Check sheet for the modelled part. Datum: model origin and axes. Units: mm. A direction names the side the tool comes from. Round coordinates to 2 decimals unless told otherwise and drop trailing zeros. Order: outer loops, then holes, each group sorted by start corner. A loop starts at its lowest first (then second) coordinate and runs counter-clockwise, first axis right, second up. Notation, with made-up numbers: M 58.25,73.25 L 84.25,73.25 A18 cw 84.25,82.25 Z; hole C 44.5,23.5 d1. An arc over 180 degrees is marked long. One line per item, written item: value. Start each with the question number.
(1) Cross-section at D-D, the plane y = -17. Enter the section's corners in (x, z), and give its area (3 significant figures).
(2) Release check for a two-part mould opening along X. For faces 3 (the face through (-13, -4, -7)), 4 (the face through (0, 17.75, -7)), 5 (the face through (20, 0, 2)) record: released by +X, released by -X, zero draft, split by the parting line, or undercut.
(3) Depth check by flat-ended pin: pin 1 Ø4 at (x, z) = (-1.5, -7) entering from +Y; pin 2 Ø3.5 at (y, z) = (-8.5, -9.5) entering from +X; pin 3 Ø2 at (y, z) = (2.5, -7.5) entering from -X. Enter the tip coordinate at first touch or a pass-through.
(4) Cross-section at C-C, the plane x = -1. Enter the section's corners in (y, z), and give its area (3 significant figures).
(5) Cross-section at A-A, the plane z = -6.5. Enter the section's corners in (x, y), and give its area (3 significant figures).
(6) Access from +Z, -Z, +X, -X, +Y, -Y to the whole of each face (thin tool, end or side, straight path). Record for faces 1 (the face through (10, 15.25, -7)), 2 (the face through (19.43, -19.4, 1.97)).
(7) Thickness scan on L1, parallel to Y at x = 15, z = -9.5; L2, parallel to X at y = -6, z = -1.5. Record the ranges inside material, lowest first.
(8) Cross-section at B-B, the plane y = 7.5. Enter the section's corners in (x, z), and give its area (3 significant figures).
from build123d import *

# Parameters (mm, degrees)
P_IDAT_VYSUNUT_M1_DEPTH = 4
SKICA2_W                = 30.5
SKICA2_H                = 30.5
SKICA2_W_2              = 4
SKICA2_H_2              = 4
P_IDAT_VYSUNUT_M2_DEPTH = 15


with BuildPart() as part:
    # Skica1 → Přidat vysunutím1 (new body)
    with BuildSketch(Plane.XY):
        with BuildLine():
            Line((-18, 20), (18, 20))
            ThreePointArc((18, 20), (19.414213562, 19.414213562), (20, 18))
            Line((20, 18), (20, -18))
            ThreePointArc((20, -18), (19.414213562, -19.414213562), (18, -20))
            Line((18, -20), (-18, -20))
            ThreePointArc((-18, -20), (-19.414213562, -19.414213562), (-20, -18))
            Line((-20, -18), (-20, 18))
            ThreePointArc((-20, 18), (-19.414213562, 19.414213562), (-18, 20))
        make_face()
    extrude(amount=P_IDAT_VYSUNUT_M1_DEPTH)

    # Skica2 → Přidat vysunutím2 (add)
    with BuildSketch(Plane(origin=(0, 0, 0), x_dir=(-1, 0, 0), z_dir=(0, 0, -1))):
        with BuildLine():
            ThreePointArc((-17.75, 15.75), (-17.164213562, 17.164213562), (-15.75, 17.75))
            Line((-15.75, 17.75), (15.75, 17.75))
            ThreePointArc((15.75, 17.75), (17.164213562, 17.164213562), (17.75, 15.75))
            Line((17.75, 15.75), (17.75, -15.75))
            ThreePointArc((17.75, -15.75), (17.164213562, -17.164213562), (15.75, -17.75))
            Line((15.75, -17.75), (-15.75, -17.75))
            ThreePointArc((-15.75, -17.75), (-17.164213562, -17.164213562), (-17.75, -15.75))
            Line((-17.75, -15.75), (-17.75, 15.75))
        make_face()
        Rectangle(SKICA2_W, SKICA2_H, mode=Mode.SUBTRACT)
        with Locations((-2, 13.25)):
            Rectangle(SKICA2_W_2, SKICA2_H_2)
        with Locations((2, 13.25)):
            Rectangle(SKICA2_W_2, SKICA2_H_2)
        with Locations((13.25, 2)):
            Rectangle(SKICA2_W_2, SKICA2_H_2)
        with Locations((13.25, -2)):
            Rectangle(SKICA2_W_2, SKICA2_H_2)
        with Locations((2, -13.25)):
            Rectangle(SKICA2_W_2, SKICA2_H_2)
        with Locations((-2, -13.25)):
            Rectangle(SKICA2_W_2, SKICA2_H_2)
        with Locations((-13.25, 2)):
            Rectangle(SKICA2_W_2, SKICA2_H_2)
        with Locations((-13.25, -2)):
            Rectangle(SKICA2_W_2, SKICA2_H_2)
    extrude(amount=P_IDAT_VYSUNUT_M2_DEPTH)


solid = part.part
Values found:
1. outline: M -20,0 L -17.31,0 L -17.31,-15 L 17.31,-15 L 17.31,0 L 20,0 L 20,4 L -20,4 Z
1. area: 679 mm^2
2. face 3: undercut
2. face 4: zero draft
2. face 5: released by +X
3. pin 1: y = 17.75
3. pin 2: x = 17.75
3. pin 3: x = -17.75
4. outline: M -20,0 L -17.75,0 L -17.75,-15 L -11.25,-15 L -11.25,0 L 11.25,0 L 11.25,-15 L 17.75,-15 L 17.75,0 L 20,0 L 20,4 L -20,4 Z
4. area: 355 mm^2
5. outline: M -17.75,-15.75 A2 ccw -15.75,-17.75 L 15.75,-17.75 A2 ccw 17.75,-15.75 L 17.75,15.75 A2 ccw 15.75,17.75 L -15.75,17.75 A2 ccw -17.75,15.75 Z; hole M -15.25,-15.25 L -4,-15.25 L -4,-11.25 L 4,-11.25 L 4,-15.25 L 15.25,-15.25 L 15.25,-4 L 11.25,-4 L 11.25,4 L 15.25,4 L 15.25,15.25 L 4,15.25 L 4,11.25 L -4,11.25 L -4,15.25 L -15.25,15.25 L -15.25,4 L -11.25,4 L -11.25,-4 L -15.25,-4 Z
5. area: 455 mm^2
6. face 1: -Z
6. face 2: +Z, -Z, +X, -Y
7. L1: -17.75 to -15.25, -4 to 4, 15.25 to 17.75
7. L2: -17.75 to -15.25, 15.25 to 17.75
8. outline: M -20,0 L -17.75,0 L -17.75,-15 L -15.25,-15 L -15.25,0 L 15.25,0 L 15.25,-15 L 17.75,-15 L 17.75,0 L 20,0 L 20,4 L -20,4 Z
8. area: 235 mm^2
